from build123d import *

# Parameters (mm, degrees)
SKETCH1_R           = 2.413
BOSS_EXTRUDE1_DEPTH = 3.175


with BuildPart() as part:
    # Sketch1 → Boss-Extrude1 (new body)
    with BuildSketch(Plane.XY):
        Polygon((0, 0), (33.02, 0), (33.02, 25.4), (63.5, 25.4), (63.5, 304.8), (47.625, 304.8), (0, 25.4), align=None)
        with Locations((12.7, 12.7)):
            Circle(SKETCH1_R, mode=Mode.SUBTRACT)
        with Locations((25.4, 12.7)):
            Circle(SKETCH1_R, mode=Mode.SUBTRACT)
        with Locations((60.325, 63.5)):
            Circle(SKETCH1_R, mode=Mode.SUBTRACT)
        with Locations((60.325, 114.3)):
            Circle(SKETCH1_R, mode=Mode.SUBTRACT)
        with Locations((60.325, 165.1)):
            Circle(SKETCH1_R, mode=Mode.SUBTRACT)
        with Locations((60.325, 215.9)):
            Circle(SKETCH1_R, mode=Mode.SUBTRACT)
        with Locations((60.325, 266.7)):
            Circle(SKETCH1_R, mode=Mode.SUBTRACT)
        Polygon((47.625, 205.909333333), (47.625, 45.72), (20.32, 45.72), align=None, mode=Mode.SUBTRACT)
    extrude(amount=BOSS_EXTRUDE1_DEPTH)


solid = part.part
Work out the finished part from the listing and answer in its coordinate system (mm). A direction names the side the tool comes from. Give positions to 0.01 mm unless a question says otherwise; leave off trailing zeros. Loops run counter-clockwise (first coordinate to the right, second up) from the corner with the lowest first, then second, coordinate; pieces in that order, holes last. Notation, with made-up numbers: (40, 19) -> (79, 19) arc R13 cw to (79, 37) -> close; hole circle Ø7 at (-35.5, -25.5). An arc over 180 degrees is marked (long way). Use a Markdown table: item, result. Add a question column.
1. Determine the mould class of faces 1 (the flat face through (38, 155, 0)), 2 (the cylindrical face through (12.177, 10.344, 1.565)), 3 (the flat face through (24.146, 167.056, 1.565)) for opening direction X: released by +X, released by -X, zero draft, split by the parting line, or undercut.
2. Section A-A on z = 0.6 is taken. State how many separate pieces and enclosed holes the cut face has, and give its area (3 significant figures).
3. Find the intervals of material crossed by probe 1 along Y at (x, z) = (61, 0.4); probe 2 along X at (y, z) = (61.5, 0.7) (3 decimals); probe 3 along X at (y, z) = (188, 2.4) (3 decimals), in increasing order.
4. A flat-ended cylindrical pin translates along its axis: pin 1 Ø1.6 at (x, z) = (53, 2) entering from -Y. Find the tip coordinate at first contact, or state that the pin passes through.
5. For faces 4 (the flat face through (33.78, 124.69, 1.57)), 5 (the flat face through (38, 155, 3.175)), determine the directions among +Z, -Z, +X, -X, +Y, -Y from which every point of the face is accessible in a straight line to the end or side of a thin tool.
6. Section B-B on x = 40.5 is taken. Determine the outline of the cut face in (y, z) (3 decimals).
7. Section C-C on y = 101.5 is taken. Determine the outline of the cut face in (x, z) (3 decimals).
8. Section D-D on x = 53 is taken. Determine the outline of the cut face in (y, z) (3 decimals), and give its area (3 significant figures).
Results below:
| question | item | result |
|---|---|---|
| 1 | face 1 | zero draft |
| 1 | face 2 | undercut |
| 1 | face 3 | released by -X |
| 2 | separate pieces | 1 |
| 2 | enclosed holes | 8 |
| 2 | area | 9,610 mm^2 |
| 3 | probe 1 | y = 25.4 to 61.18, 65.82 to 111.98, 116.62 to 162.78, 167.42 to 213.58, 218.22 to 264.38, 269.02 to 304.8 |
| 3 | probe 2 | x = 6.153 to 23.01, 47.625 to 58.975, 61.675 to 63.5 |
| 3 | probe 3 | x = 27.716 to 44.572, 47.625 to 63.5 |
| 4 | pin 1 | stops at y = 25.4 |
| 5 | face 4 | +Z, -Z |
| 5 | face 5 | +Z, +X, -X, +Y, -Y |
| 6 | outline | (25.4, 0) -> (45.72, 0) -> (45.72, 3.175) -> (25.4, 3.175) -> close; (164.109, 0) -> (263, 0) -> (263, 3.175) -> (164.109, 3.175) -> close |
| 7 | outline | (12.972, 0) -> (29.828, 0) -> (29.828, 3.175) -> (12.972, 3.175) -> close; (47.625, 0) -> (63.5, 0) -> (63.5, 3.175) -> (47.625, 3.175) -> close |
| 8 | outline | (25.4, 0) -> (304.8, 0) -> (304.8, 3.175) -> (25.4, 3.175) -> close |
| 8 | area | 887 mm^2 |
